from build123d import *

# Parameters (mm, degrees)
BASPROSKE_W                  = 12.5
BASPROSKE_H                  = 17.5
TOOTHCUT_DEPTH               = 28.726341266
TEETHCUTS_COUNT              = 12
TEETHCUTS_ANGLE              = 330
BORSKE_R                     = 0.75
BORE_DEPTH                   = 50.0000508
ENL_V_MAT_EXTRU_2_DEPTH      = 10
ENL_V_MAT_EXTRU_2_DEPTH_BACK = 60
ESQUISSE1_R                  = 5
ESQUISSE2_R                  = 8.5
BOSS_EXTRU_1_DEPTH           = 10


with BuildPart() as part:
    # BasProSke → Base-Revolve (revolve)
    with BuildSketch(Plane(origin=(0, 0, 0), x_dir=(1, 0, 0), z_dir=(0, 1, 0)), mode=Mode.PRIVATE) as base_revolve_sk:
        with Locations((6.25, 8.75)):
            Rectangle(BASPROSKE_W, BASPROSKE_H)
    revolve(base_revolve_sk.sketch.rotate(Axis((-10, 0, 0), (1, 0, 0)), 180), axis=Axis((-10, 0, 0), (1, 0, 0)))

    # TooCutSke → ToothCut (cut, through all)
    with BuildSketch(Plane(origin=(0, 0, 0), x_dir=(0, 0, -1), z_dir=(1, 0, 0))):
        with BuildLine():
            ThreePointArc((1.612970859, 11.763936459), (0, 11.874), (-1.612970859, 11.763936459))
            ThreePointArc((-1.612970859, 11.763936459), (-2.052105863, 14.718225349), (-3.861172246, 17.094765107))
            ThreePointArc((-3.861172246, 17.094765107), (0, 17.5254), (3.861172246, 17.094765107))
            ThreePointArc((3.861172246, 17.094765107), (2.052105863, 14.718225349), (1.612970859, 11.763936459))
        make_face()
    toothcut = extrude(amount=TOOTHCUT_DEPTH, mode=Mode.SUBTRACT)

    # TeethCuts: ToothCut ×12 about axis
    teethcuts_axis = Axis((-10, 0, 0), (1, 0, 0))
    for i in range(1, TEETHCUTS_COUNT):
        add(toothcut.rotate(teethcuts_axis, i * TEETHCUTS_ANGLE / (TEETHCUTS_COUNT - 1)), mode=Mode.SUBTRACT)

    # BorSke → Bore (cut, symmetric)
    with BuildSketch(Plane(origin=(0, 0, 0), x_dir=(0, 0, -1), z_dir=(1, 0, 0))):
        with Locations(Location((0, 0, 0), (0, 0, 180))):
            Circle(BORSKE_R)
    extrude(amount=BORE_DEPTH, both=True, mode=Mode.SUBTRACT)

    # Esquisse1 → Enlèv. mat.-Extru.2 (cut, two sides: drawn at the far end of the back side and taken through both)
    with BuildSketch(Plane(origin=(12.5, 0, 0), x_dir=(0, 0, -1), z_dir=(1, 0, 0)).offset(-ENL_V_MAT_EXTRU_2_DEPTH_BACK)):
        with Locations(Location((0, 0, 0), (0, 0, 180))):
            Circle(ESQUISSE1_R)
    extrude(amount=ENL_V_MAT_EXTRU_2_DEPTH + ENL_V_MAT_EXTRU_2_DEPTH_BACK, mode=Mode.SUBTRACT)

    # Esquisse2 → Boss.-Extru.1 (add)
    with BuildSketch(Plane(origin=(12.5, 0, 0), x_dir=(0, 0, -1), z_dir=(1, 0, 0))):
        with Locations(Location((0, 0, 0), (0, 0, 180))):
            Circle(ESQUISSE2_R)
    extrude(amount=BOSS_EXTRU_1_DEPTH)


solid = part.part
Can you work these out from the model? Positions are in its coordinate system, mm. A direction names the side the tool comes from. Give positions to 0.01 mm unless a question says otherwise; leave off trailing zeros. Loops run counter-clockwise (first coordinate to the right, second up) from the corner with the lowest first, then second, coordinate; pieces in that order, holes last. Notation, with made-up numbers: M 42,79.5 L 64,79.5 A31 ccw 64,109.5 Z; hole C 15,50 d8. An arc over 180 degrees is marked long. One line per item, written item: value. Start each with the question number.
1) If we section it at C-C, the plane x = 14.25: Write out the boundary of the cut face in (y, z).
2) If we section it at D-D, the plane y = 13.5: Write out the boundary of the cut face in (x, z).
3) Thinking about a two-plate mould opening in Z: for faces 4 (the face through (6.34, 12.38, 12.37)), 5 (the face through (6.16, -11.74, 9.16)), 6 (the face through (6.34, 12.37, -12.38)), which applies, +Z half, -Z half, draft (parallel to the pull), parting line (faces both ways), or undercut?
4) If we section it at A-A, the plane z = 0: Write out the boundary of the cut face in (x, y).
5) If I drill on line 1 (Z direction, x = 2, y = -10); line 2 (Z direction, x = 1.5, y = 11.5), over which ranges is the centre line in solid material (lowest first)? Write a range as [from, to].
6) I'm going to push flat-ended pins straight in: pin 1 (4 mm diameter, centred on y = 0, z = 6, fed in from -X); pin 2 (4 mm diameter, centred on x = 3, z = -13, fed in from +Y); pin 3 (3 mm diameter, centred on x = 19.5, z = 7, fed in from +Y); pin 4 (4 mm diameter, centred on y = 9.5, z = -10, fed in from +X). Where does each tip first touch, or does it pass through?
7) On a 3-axis mill with a long thin cutter (end or side, diameter ignored), from which of +Z, -Z, +X, -X, +Y, -Y can I reach the whole of each face in a straight line? I mean faces 1 (the face through (6.16, 9.16, 11.74)), 2 (the face through (6.338, 4.52, -16.906)), 3 (the face through (6, 0, -5)). Say none if no direction works.
Completed:
1. outline: C 0,0 d17
2. outline: M 0,-5.54 L 12.5,-5.54 L 12.5,-1.68 L 0,-1.68 Z; M 0,1.68 L 12.5,1.68 L 12.5,5.54 L 0,5.54 Z
3. face 4: +Z half
3. face 5: undercut
3. face 6: -Z half
4. outline: M 0,-11.87 L 12.5,-11.87 L 12.5,-8.5 L 22.5,-8.5 L 22.5,8.5 L 12.5,8.5 L 12.5,11.87 L 0,11.87 L 0,5 L 12.5,5 L 12.5,-5 L 0,-5 Z
5. line 1: z = [-12.27, -7.6], [-6.4, 6.4], [7.6, 12.27]
5. line 2: z = [-12.8, -8.86], [-4.81, 4.81], [8.86, 12.8]
6. pin 1: stops at x = 0
6. pin 2: stops at y = 12.87
6. pin 3: stops at y = 6.48
6. pin 4: stops at x = 12.5
7. face 1: +Z, +X, -X
7. face 2: -Z, +X, -X, +Y
7. face 3: -X
